The model under review builds one solid part; all positions refer to its coordinate system, in mm. A direction names the side the tool comes from. Coordinates: 2 decimals unless noted, no trailing zeros. Write each loop counter-clockwise with the first axis right and the second up, starting at its lowest first coordinate (ties: lowest second). Pieces come first, ordered by that corner, then holes. Notation, with made-up numbers: (-32, 22.5) - (-28, 22.5) arc R10 cw to (-28, 31.5) - close; hole circle Ø11 at (-31, 24.5). An arc over 180 degrees is marked (long way). Put each result on its own line as item: value.
Autodesk Inventor part; units mm, degrees
ref_plane "YZ Plane" through (0, 0, 0) normal (1, 0, 0) x (0, 1, 0)
ref_plane "XZ Plane" through (0, 0, 0) normal (0, 1, 0) x (-1, 0, 0)
ref_plane "XY Plane" through (0, 0, 0) normal (0, 0, 1) x (1, 0, 0)
sketch "Esboço1" plane through (0, 0, 0) normal (0, 0, 1) x (1, 0, 0)
  line L0 (-90, -70) -> (70, -70)
  line L1 (70, -70) -> (70, 70)
  line L2 (70, 70) -> (-90, 70)
  line L3 (-90, 70) -> (-90, -70)
  circle A0 centre (0, 0) radius 52.5
  point P0 (70, 0)
  dimension "d0" = 140
  dimension "d1" = 160
  dimension "d2" = 70
  dimension "d3" = 105
extrude "Extrusão1" add sketch "Esboço1" along normal blind 3
sketch "Esboço2" plane through (0, 0, 3) normal (0, 0, 1) x (1, 0, 0)
  line L0 (70, -70) -> (70, 70)
  line L1 (70, 70) -> (-90, 70)
  line L2 (-90, -70) -> (70, -70)
  circle A0 centre (-55, 55) radius 8
  circle A1 centre (55, 55) radius 8
  circle A2 centre (55, -55) radius 8
  circle A3 centre (-55, -55) radius 8
  dimension "d6" = 16
  dimension "d7" = 15
  dimension "d8" = 15
  dimension "d9" = 15
  dimension "d10" = 15
  dimension "d11" = 110
extrude "Extrusão2" cut sketch "Esboço2" against normal up to next
sketch "Esboço3" plane through (0, 0, 3) normal (0, 0, 1) x (1, 0, 0)
  circle A0 centre (0, 0) radius 52.5
  arc A1 (-65, 5) -> (-65, -5) centre (-65, 0) ccw
  line L0 (-65, 5) -> (-45, 5)
  line L1 (-45, 5) -> (-45, -5)
  line L2 (-45, -5) -> (-65, -5)
  dimension "d14" = 65
  dimension "d15" = 5
  dimension "d16" = 20
extrude "Extrusão3" cut sketch "Esboço3" against normal up to next contours L0 L1 L2 A0 | A0 L2 A1 L0 picked at (-47.4912, 0.5563)
fillet "Arredondamento1" radius 15 4 edges at (70, 70, 1.5) (70, -70, 1.5) (-90, -70, 1.5) (-90, 70, 1.5)
1. The part is to be moulded in two halves that separate along X. For faces 1 (the flat face through (-47, 32, 3)), 2 (the cylindrical face through (-56.041, -47.068, 1.521)), 3 (the cylindrical face through (65.49, -65.72, 1.52)), 4 (the cylindrical face through (-85.49, 65.72, 1.52)), say which applies: +X half, -X half, draft (parallel to the pull), parting line (faces both ways), or undercut.
Determined:
face 1: draft
face 2: undercut
face 3: +X half
face 4: -X half
2. Consider section D-D on y = -58. State the section outline as (x, z) points, plus the area to 3 significant figures.
Determined:
outline: (-89.7, 0) - (-62.42, 0) - (-62.42, 3) - (-89.7, 3) - close; (-47.58, 0) - (47.58, 0) - (47.58, 3) - (-47.58, 3) - close; (62.42, 0) - (69.7, 0) - (69.7, 3) - (62.42, 3) - close
area: 389 mm^2
3. Consider section C-C on x = 0. State the section outline as (y, z) points, plus the area to 3 significant figures.
Determined:
outline: (-70, 0) - (-52.5, 0) - (-52.5, 3) - (-70, 3) - close; (52.5, 0) - (70, 0) - (70, 3) - (52.5, 3) - close
area: 105 mm^2
4. For pin 1 Ø12 at (x, y) = (-41.5, 16.5) entering from -Z, flat-tipped, find the tip position at first contact; note if it passes through.
Determined:
pin 1: passes through
5. Consider section A-A on x = -55. State the section outline as (y, z) points.
Determined:
outline: (-70, 0) - (-63, 0) - (-63, 3) - (-70, 3) - close; (-47, 0) - (-5, 0) - (-5, 3) - (-47, 3) - close; (5, 0) - (47, 0) - (47, 3) - (5, 3) - close; (63, 0) - (70, 0) - (70, 3) - (63, 3) - close
6. Consider section B-B on z = 1.2. State the section outline as (x, y) points, plus the area to 3 significant figures.
Determined:
outline: (-90, -55) arc R15 ccw to (-75, -70) - (55, -70) arc R15 ccw to (70, -55) - (70, 55) arc R15 ccw to (55, 70) - (-75, 70) arc R15 ccw to (-90, 55) - close; hole (-65, -5) - (-52.26, -5) arc R52.5 ccw (long way) to (-52.26, 5) - (-65, 5) arc R5 ccw to start; hole circle Ø16 at (-55, -55); hole circle Ø16 at (-55, 55); hole circle Ø16 at (55, -55); hole circle Ø16 at (55, 55)
area: 12,600 mm^2
7. Machinability: for faces 5 (the cylindrical face through (-70, 0, 2)), 6 (the cylindrical face through (-85.72, -65.49, 1.52)), which of the approach directions +Z, -Z, +X, -X, +Y, -Y give a long, thin tool a straight path to every point of the face, cutting with its end or side? Answer none if there is none.
Determined:
face 5: +Z, -Z
face 6: +Z, -Z, -X, -Y
8. To check wall thickness, follow probe 1 along Y at (x, z) = (55, 0.8); probe 2 along Y at (x, z) = (-59.5, 0.4); probe 3 along Y at (x, z) = (57, 2.75). State the ranges of each line that lie inside material, in increasing order.
Determined:
probe 1: y = -70 to -63, -47 to 47, 63 to 70
probe 2: y = -70 to -61.61, -48.39 to -5, 5 to 48.39, 61.61 to 70
probe 3: y = -69.87 to -62.75, -47.25 to 47.25, 62.75 to 69.87
